Source: CAD feature listing. Evaluate the final solid. Frame: model axes, mm. A direction names the side the tool comes from. Round coordinates to 2 decimals unless told otherwise and drop trailing zeros. Write each loop counter-clockwise with the first axis right and the second up, starting at its lowest first coordinate (ties: lowest second). Pieces come first, ordered by that corner, then holes. Notation, with made-up numbers: M -23,56.5 L 6,56.5 A17 ccw 6,84.5 Z; hole C -9.5,5 d1. An arc over 180 degrees is marked long. Use a Markdown table: item, result.
```python
from build123d import *

# Parameters (mm, degrees)
BOSS_EXTRUDE7_DEPTH  = 10
SKETCH1_11_R         = 5.01447977
BOSS_EXTRUDE8_DEPTH  = 12.5
SKETCH2_R            = 3.5
BOSS_EXTRUDE9_DEPTH  = 2.5
SKETCH3_R            = 1
BOSS_EXTRUDE10_DEPTH = 2.5


with BuildPart() as part:
    # Sketch1 → Boss-Extrude7 (new body)
    with BuildSketch(Plane(origin=(0, 0, 0), x_dir=(1, 0, 0), z_dir=(0, 1, 0))):
        with BuildLine():
            Line((-5, 46.203703704), (-5, -153.415497967))
            ThreePointArc((-5, -153.415497967), (0, -148.781816526), (5, -153.415497967))
            Line((5, -153.415497967), (5, 46.203703704))
            ThreePointArc((5, 46.203703704), (0, 51.203703704), (-5, 46.203703704))
        make_face()
        with BuildLine():
            ThreePointArc((-2.5, -37.014405443), (0, -34.514405443), (2.5, -37.014405443))
            Line((2.5, -37.014405443), (2.5, -143.90389726))
            ThreePointArc((2.5, -143.90389726), (0, -146.40389726), (-2.5, -143.90389726))
            Line((-2.5, -143.90389726), (-2.5, -37.014405443))
        make_face(mode=Mode.SUBTRACT)
        with BuildLine():
            ThreePointArc((-2.5, 46.203703704), (0, 48.703703704), (2.5, 46.203703704))
            Line((2.5, 46.203703704), (2.5, -17.887410681))
            ThreePointArc((2.5, -17.887410681), (0, -20.387410681), (-2.5, -17.887410681))
            Line((-2.5, -17.887410681), (-2.5, 46.203703704))
        make_face(mode=Mode.SUBTRACT)
    extrude(amount=BOSS_EXTRUDE7_DEPTH)

    # Sketch1_11 → Boss-Extrude8 (add)
    with BuildSketch(Plane(origin=(0, 0, 0), x_dir=(1, 0, 0), z_dir=(0, 1, 0))):
        with Locations(Location((0, -153.796296296, 0), (0, 0, 4.355219889))):
            Circle(SKETCH1_11_R)
    extrude(amount=BOSS_EXTRUDE8_DEPTH)

    # Sketch2 → Boss-Extrude9 (add)
    with BuildSketch(Plane(origin=(0, 12.5, 0), x_dir=(1, 0, 0), z_dir=(0, 1, 0))):
        with Locations(Location((0, -153.796296296, 0), (0, 0, 270))):
            Circle(SKETCH2_R)
    extrude(amount=BOSS_EXTRUDE9_DEPTH)

    # Sketch3 → Boss-Extrude10 (add)
    with BuildSketch(Plane(origin=(0, 15, 0), x_dir=(1, 0, 0), z_dir=(0, 1, 0))):
        with Locations(Location((0, -153.796296296, 0), (0, 0, 270))):
            Circle(SKETCH3_R)
    extrude(amount=BOSS_EXTRUDE10_DEPTH)


solid = part.part
```
Q1. Line query: L1, parallel to X at y = 9.75, z = 93.5; L2, parallel to Z at x = 0.75, y = 4.5; L3, parallel to Z at x = 2, y = 5. Output: solid intervals per line, ascending.
Results are:
| item | result |
|---|---|
| L1 | -5 to -2.5, 2.5 to 5 |
| L2 | -51.15 to -48.59, 20.27 to 34.63, 146.29 to 158.75 |
| L3 | -50.79 to -47.7, 19.39 to 35.51, 145.4 to 158.39 |
Q2. Mould query, pull axis Z, two halves, no side actions, for faces 1 (the cylindrical face through (0.11, 4.93, -51.202)), 2 (the flat face through (-5, 5, 52)), 3 (the flat face through (-2.5, 5, 91)). Classes: +Z half, -Z half, draft (parallel to the pull), parting line (faces both ways), or undercut.
Results are:
| item | result |
|---|---|
| face 1 | -Z half |
| face 2 | draft |
| face 3 | undercut |
Q3. Section B-B on y = 3.25. Return loops of the section in (x, z).
Results are:
| item | result |
|---|---|
| outline | M -5,-46.2 A5 ccw 5,-46.2 L 5,153.42 A5.01 ccw long -5,153.42 Z; hole M -2.5,-46.2 A2.5 ccw 2.5,-46.2 L 2.5,17.89 A2.5 ccw -2.5,17.89 Z; hole M -2.5,37.01 A2.5 ccw 2.5,37.01 L 2.5,143.9 A2.5 ccw -2.5,143.9 Z |
Q4. Section A-A on z = 116. Return loops of the section in (x, y), plus the area to 3 significant figures.
Results are:
| item | result |
|---|---|
| outline | M -5,0 L -2.5,0 L -2.5,10 L -5,10 Z; M 2.5,0 L 5,0 L 5,10 L 2.5,10 Z |
| area | 50.0 mm^2 |
Q5. Reachability of faces 4 (the flat face through (-2.5, 5, -14)), 5 (the cylindrical face through (-1.34, 13.73, 157.03)), 6 (the flat face through (4, 0, 61)) from +Z, -Z, +X, -X, +Y, -Y: full face, straight path, thin tool, end or side. Return the list, or none.
Results are:
| item | result |
|---|---|
| face 4 | +Y, -Y |
| face 5 | +Y |
| face 6 | +Z, -Z, +X, -X, -Y |
Q6. First-contact query: pin 1 Ø4 at (x, z) = (-2.5, -15) entering from +Y; pin 2 Ø4 at (y, z) = (5.5, 100.5) entering from -X; pin 3 Ø8 at (y, z) = (5, 1) entering from +X. Flat tips, straight axial feed; report the tip coordinate or a pass-through.
Results are:
| item | result |
|---|---|
| pin 1 | y = 10 |
| pin 2 | x = -5 |
| pin 3 | x = 5 |
